Model file for the job. Use its own axes, mm. A direction names the side the tool comes from. Coordinates: 2 decimals unless noted, no trailing zeros. Write each loop counter-clockwise with the first axis right and the second up, starting at its lowest first coordinate (ties: lowest second). Pieces come first, ordered by that corner, then holes. Notation, with made-up numbers: (-26, -25) -> (-7, -25) arc R11 cw to (-7, -15) -> close; hole circle Ø1 at (-40, 41). An arc over 180 degrees is marked (long way). Answer as a JSON object with one key per item and string values. Group by question number.
from build123d import *

# Parameters (mm, degrees)
SKETCH1_W                      = 29
SKETCH1_H                      = 6
BOSS_EXTRUDE1_DEPTH            = 10
SKETCH5_W                      = 13.5
SKETCH5_H                      = 3
BOSS_EXTRUDE2_DEPTH            = 8
CBORE_FOR_M3_SHCS1_D           = 3.4
CBORE_FOR_M3_SHCS1_CBORE_D     = 6.5
CBORE_FOR_M3_SHCS1_CBORE_DEPTH = 3
CHAMFER1_SIZE                  = 3


with BuildPart() as part:
    # Sketch1 → Boss-Extrude1 (new body)
    with BuildSketch(Plane.XY):
        Rectangle(SKETCH1_W, SKETCH1_H)
    extrude(amount=BOSS_EXTRUDE1_DEPTH)

    # Sketch5 → Boss-Extrude2 (add)
    with BuildSketch(Plane.XY.offset(10)):
        with Locations((0, 1.5)):
            Rectangle(SKETCH5_W, SKETCH5_H)
    extrude(amount=BOSS_EXTRUDE2_DEPTH)

    # CBORE for M3 SHCS1 (through all)
    with Locations(Plane.XY.offset(10)):
        with Locations((-10, 0), (10, 0)):
            CounterBoreHole(CBORE_FOR_M3_SHCS1_D / 2, CBORE_FOR_M3_SHCS1_CBORE_D / 2, CBORE_FOR_M3_SHCS1_CBORE_DEPTH)

    # Chamfer1
    chamfer1_edges = [part.edges().sort_by_distance(p)[0] for p in [
        (0, 0, 18),
    ]]
    chamfer(chamfer1_edges, length=CHAMFER1_SIZE - 0.0001)  # a hair under: the kernel refuses the full size


solid = part.part
(1) Pull direction Y, two halves, no side cores. Call faces 1 (the face through (-13.25, 0.05, 8.52)), 2 (the face through (0, -3, 5)), 3 (the face through (6.75, 1, 13)): released by +Y, released by -Y, zero draft, split by the parting line, or undercut.
(2) Pin check, flat tips, straight feed: pin 1 (1 mm diameter, centred on x = 7.5, y = 1, fed in from +Z); pin 2 (2 mm diameter, centred on y = 1, z = 15.5, fed in from -X); pin 3 (2.5 mm diameter, centred on x = -4, y = -1, fed in from +Z). Stop position of each tip, or through.
(3) Wall check: probe 1 along X at (y, z) = (-1.4, 6); probe 2 along Y at (x, z) = (-10, 5.75); probe 3 along X at (y, z) = (2.2, 12). Give the ranges that are in metal, low to high.
(4) 3-axis set-ups, long thin cutter, end or side, ignore diameter. For faces 4 (the face through (0, -1, 10)), 5 (the face through (14, 0, 10)), 6 (the face through (-6.75, 1, 13)), 7 (the face through (8.43, -0.65, 3.45)), 8 (the face through (6.75, 0.05, 8.52)): which of +Z, -Z, +X, -X, +Y, -Y reach the whole face in a straight line?
(5) Cut at C-C on y = -0.8. List the corners of the cut face in (x, z), plus the area to 3 significant figures.
(6) Cut at B-B on z = 9.5. List the corners of the cut face in (x, y), plus the area to 3 significant figures.
(7) Cut at A-A on x = 10. List the corners of the cut face in (y, z), plus the area to 3 significant figures.
Results found:
{
 "1": {"face 1": "undercut", "face 2": "released by -Y", "face 3": "zero draft"},
 "2": {"pin 1": "stops at z = 7", "pin 2": "stops at x = -6.75", "pin 3": "stops at z = 15.25"},
 "3": {"probe 1": "x = -14.5 to -10.96, -9.04 to 9.04, 10.96 to 14.5", "probe 2": "y = -3 to -1.7, 1.7 to 3", "probe 3": "x = -6.75 to 6.75"},
 "4": {"face 4": "+Z, +X, -X, -Y", "face 5": "+Z, +X, +Y, -Y", "face 6": "+Z, -X, +Y, -Y", "face 7": "+Z, -Z", "face 8": "+Z"},
 "5": {"outline": "(-14.5, 0) -> (-11.5, 0) -> (-11.5, 7) -> (-13.15, 7) -> (-13.15, 10) -> (-14.5, 10) -> close; (-8.5, 0) -> (8.5, 0) -> (8.5, 7) -> (6.85, 7) -> (6.85, 10) -> (-6.85, 10) -> (-6.85, 7) -> (-8.5, 7) -> close; (11.5, 0) -> (14.5, 0) -> (14.5, 10) -> (13.15, 10) -> (13.15, 7) -> (11.5, 7) -> close", "area": "210 mm²"},
 "6": {"outline": "(-14.5, -3) -> (-11.25, -3) arc R3.25 cw to (-11.25, 3) -> (-14.5, 3) -> close; (-8.75, -3) -> (8.75, -3) arc R3.25 cw to (8.75, 3) -> (-8.75, 3) arc R3.25 cw to start; (11.25, -3) -> (14.5, -3) -> (14.5, 3) -> (11.25, 3) arc R3.25 cw to start", "area": "109 mm²"},
 "7": {"outline": "(-3, 0) -> (-1.7, 0) -> (-1.7, 7) -> (-3, 7) -> close; (1.7, 0) -> (3, 0) -> (3, 7) -> (1.7, 7) -> close", "area": "18.2 mm²"}
}
